Build history of the part. All positions in model axes, mm. Face numbers are marked on the shaded views. Give positions to 0.01 mm unless a question says otherwise; leave off trailing zeros. Write each loop counter-clockwise with the first axis right and the second up, starting at its lowest first coordinate (ties: lowest second). Pieces come first, ordered by that corner, then holes. Notation, with made-up numbers: (30, 17.5) - (75, 17.5) arc R26 cw to (75, 32.5) - close; hole circle Ø7 at (25.25, 21). An arc over 180 degrees is marked (long way). Use one line per item in the form item = value. Start each with the question number.
from build123d import *


with BuildPart() as part:
    # Esquisse1 → Révolution1 (revolve)
    with BuildSketch(Plane(origin=(0, 0, 0), x_dir=(0, 0, -1), z_dir=(1, 0, 0)), mode=Mode.PRIVATE) as r_volution1_sk:
        with BuildLine():
            Line((-6.5, 18), (6.5, 18))
            Line((6.5, 18), (6.5, 19))
            Line((6.5, 19), (7.5, 19))
            Line((7.5, 19), (7.5, 24.894778569))
            ThreePointArc((7.5, 24.894778569), (0, 26), (-7.5, 24.894778569))
            Line((-7.5, 24.894778569), (-7.5, 19))
            Line((-7.5, 19), (-6.5, 19))
            Line((-6.5, 19), (-6.5, 18))
        make_face()
    revolve(r_volution1_sk.sketch.rotate(Axis((0, 0, 2.4656375), (0, 0, -1)), 90), axis=Axis((0, 0, 2.4656375), (0, 0, -1)))


solid = part.part
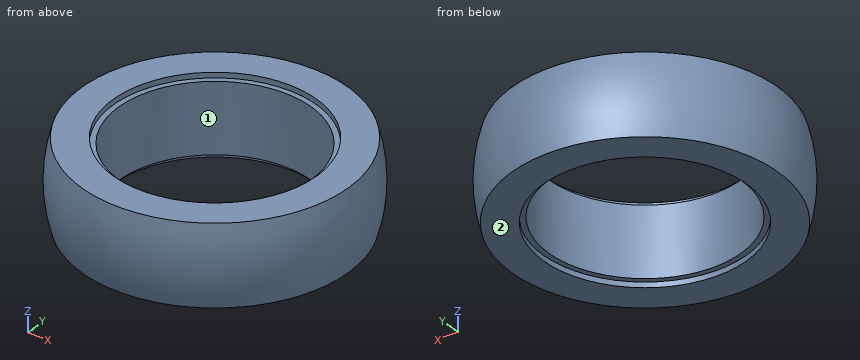
(1) Cut at A-A, the plane y = 0. Give the cut face in (x, z).
(2) Two-plate mould, pull along X, no slides. Class the marked faces 1 and 2: +X half, -X half, draft (parallel to the pull), parting line (faces both ways), or undercut.
(3) Wall check: line 1 (X direction, y = 4.5, z = 1.5); line 2 (X direction, y = 9, z = -3.5); line 3 (Y direction, x = 13, z = -5.5). Give the ranges that are in metal, low to high. Write a range as from..to.
(4) Cut at D-D, the plane y = 21.5. Give the cut face in (x, z), then the cut area to 3 significant figures.
(5) Pin check, flat tips, straight feed: pin 1 Ø3 at (x, z) = (-12, 1.5) entering from +Y; pin 2 Ø1.5 at (y, z) = (12.5, 0) entering from -X; pin 3 Ø8 at (y, z) = (4, -3) entering from -X; pin 4 Ø19 at (x, y) = (-8, 8) entering from -Z. Stop position of each tip, or through.
(6) Cut at C-C, the plane z = 0. Give the cut face in (x, y).
Solution:
q1.outline = (-24.89, -7.5) - (-19, -7.5) - (-19, -6.5) - (-18, -6.5) - (-18, 6.5) - (-19, 6.5) - (-19, 7.5) - (-24.89, 7.5) arc R26 ccw to start; (18, -6.5) - (19, -6.5) - (19, -7.5) - (24.89, -7.5) arc R26 ccw to (24.89, 7.5) - (19, 7.5) - (19, 6.5) - (18, 6.5) - close
q2.face_1 = undercut
q2.face_2 = draft
q3.line_1 = -25.56..-17.43, 17.43..25.56
q3.line_2 = -24.14..-15.59, 15.59..24.14
q3.line_3 = -21.83..-12.45, 12.45..21.83
q4.outline = (-12.55, -7.5) - (12.55, -7.5) arc R14.62 ccw to (12.55, 7.5) - (-12.55, 7.5) arc R14.62 ccw to start
q4.area = 419 mm2
q5.pin_1 = 23.74
q5.pin_2 = -23.19
q5.pin_3 = -25.98
q5.pin_4 = -7.5
q6.outline = circle Ø52 at (0, 0); hole circle Ø36 at (0, 0)
